Read the model definition and answer for the solid it produces. Units are mm, in the model's axes. Coordinates: 2 decimals unless noted, no trailing zeros. Write each loop counter-clockwise with the first axis right and the second up, starting at its lowest first coordinate (ties: lowest second). Pieces come first, ordered by that corner, then holes. Notation, with made-up numbers: (88.25, 56) - (147.25, 56) arc R10 cw to (147.25, 71) - close; hole circle Ø5 at (30, 9.5). An arc over 180 degrees is marked (long way). Return JSON: item names as keys, results as strings.
```python
from build123d import *

# Parameters (mm, degrees)
BOSS_EXTRUDE1_DEPTH   = 1.5875
F_6_CLEARANCE_HOLE1_D = 4.3053


with BuildPart() as part:
    # Sketch1 → Boss-Extrude1 (new body)
    with BuildSketch(Plane.XY):
        with BuildLine():
            Line((-23.8125, -87.076434182), (-23.8125, -36.276434182))
            ThreePointArc((-23.8125, -36.276434182), (-25.207403955, -32.908838137), (-28.575, -31.513934182))
            Line((-28.575, -31.513934182), (-79.375, -31.513934182))
            ThreePointArc((-79.375, -31.513934182), (-82.742596045, -32.908838137), (-84.1375, -36.276434182))
            Line((-84.1375, -36.276434182), (-84.1375, -87.076434182))
            ThreePointArc((-84.1375, -87.076434182), (-82.742596045, -90.444030228), (-79.375, -91.838934182))
            Line((-79.375, -91.838934182), (-28.575, -91.838934182))
            ThreePointArc((-28.575, -91.838934182), (-25.207403955, -90.444030228), (-23.8125, -87.076434182))
        make_face()
    extrude(amount=-BOSS_EXTRUDE1_DEPTH)

    # #6 Clearance Hole1 (through all)
    with Locations(Plane(origin=(0, 0, -1.5875), x_dir=(-1, 0, 0), z_dir=(0, 0, -1))):
        with Locations((30.401827682, -38.103261864), (77.548172318, -85.2496065)):
            Hole(F_6_CLEARANCE_HOLE1_D / 2)


solid = part.part
```
(1) Straight lines are drawn through the part: line 1 (Y direction, x = -77.5, z = -0.3); line 2 (X direction, y = -38, z = -0.25); line 3 (X direction, y = -40, z = -0.6). For each, find the intervals that lie inside material, in ascending order. Write a range as from..to.
Answer:
{"line 1": "-91.84..-87.4, -83.1..-31.51", "line 2": "-84.14..-32.55, -28.25..-23.81", "line 3": "-84.14..-31.42, -29.38..-23.81"}
(2) Determine the mould class of faces 1 (the face through (-54, -61, -1.588)), 2 (the face through (-28.4, -38.9, -0.8)), 3 (the face through (-25.245, -90.481, -0.783)) for opening direction Y: +Y half, -Y half, draft (parallel to the pull), parting line (faces both ways), or undercut.
Answer:
{"face 1": "draft", "face 2": "undercut", "face 3": "-Y half"}
(3) A cutting plane is placed at A-A (x = -31). Determine the outline of the cut face in (y, z).
Answer:
{"outline": "(-91.84, -1.59) - (-40.17, -1.59) - (-40.17, 0) - (-91.84, 0) - close; (-36.04, -1.59) - (-31.51, -1.59) - (-31.51, 0) - (-36.04, 0) - close"}
(4) A cutting plane is placed at B-B (y = -37). Determine the outline of the cut face in (x, z).
Answer:
{"outline": "(-84.14, -1.59) - (-32.25, -1.59) - (-32.25, 0) - (-84.14, 0) - close; (-28.55, -1.59) - (-23.81, -1.59) - (-23.81, 0) - (-28.55, 0) - close"}
